Geometry check sheet. Reference: the model listing, model coordinates, mm. Round coordinates to 2 decimals unless told otherwise and drop trailing zeros. Write each loop counter-clockwise with the first axis right and the second up, starting at its lowest first coordinate (ties: lowest second). Pieces come first, ordered by that corner, then holes. Notation, with made-up numbers: M -12,-6.5 L -1,-6.5 A14 cw -1,2.5 Z; hole C 63,-28 d8. An arc over 180 degrees is marked long. Answer in a Markdown table with one row per item. Add a question column.
from build123d import *

# Parameters (mm, degrees)
SKETCH1_R            = 84
BOSS_EXTRUDE1_DEPTH  = 10
M6_CLEARANCE_HOLE1_D = 7


with BuildPart() as part:
    # Sketch1 → Boss-Extrude1 (new body)
    with BuildSketch(Plane(origin=(0, 0, 0), x_dir=(1, 0, 0), z_dir=(0, 1, 0))):
        with Locations(Location((0, 0, 0), (0, 0, 270))):
            Circle(SKETCH1_R)
    extrude(amount=BOSS_EXTRUDE1_DEPTH)

    # M6 Clearance Hole1 (through all)
    with Locations(Plane(origin=(0, 10, -76), x_dir=(0, 0, 1), z_dir=(0, 1, 0))):
        with Locations((0, 0), (76, -76), (76, 76), (76, 25), (51, 0), (76, -25), (101, 0), (152, 0)):
            Hole(M6_CLEARANCE_HOLE1_D / 2)


solid = part.part
Item 1: Section check B-B, the plane x = 0. Record the boundary of the cut face in (y, z).
Item 2: Section check C-C, the plane y = 3. Give the number of separate pieces and of enclosed holes in the cut face, and give its area (3 significant figures).
Item 3: Section check D-D, the plane x = 76. Record the boundary of the cut face in (y, z), and give its area (3 significant figures).
Item 4: Section check A-A, the plane z = 0. Record the boundary of the cut face in (x, y), and give its area (3 significant figures).
Item 5: Mould release check, pull along X, two halves, no side actions. Record for faces 1 (the cylindrical face through (25.23, 4.93, 80.12)), 2 (the cylindrical face through (-21.53, 4.93, 0.46)), 3 (the flat face through (1, 0, -1)): +X half, -X half, draft (parallel to the pull), parting line (faces both ways), or undercut.
Item 6: Scan lines: probe 1 along Z at (x, y) = (0.5, 6.5); probe 2 along X at (y, z) = (4.75, 0); probe 3 along X at (y, z) = (6.25, -76). Record each from-to range of solid material in increasing order. Write a range as from..to.
Item 7: Gauge pin test, flat ends, axial feed: pin 1 Ø6 at (x, z) = (-23.5, 29) entering from -Y; pin 2 Ø4 at (y, z) = (1.5, 27) entering from +X; pin 3 Ø1.5 at (y, z) = (6, 35) entering from -X. Record the tip position at first contact, or that the pin passes through.
Result sheet:
| question | item | result |
|---|---|---|
| 1 | outline | M 0,-84 L 10,-84 L 10,-79.5 L 0,-79.5 Z; M 0,-72.5 L 10,-72.5 L 10,-28.5 L 0,-28.5 Z; M 0,-21.5 L 10,-21.5 L 10,21.5 L 0,21.5 Z; M 0,28.5 L 10,28.5 L 10,72.5 L 0,72.5 Z; M 0,79.5 L 10,79.5 L 10,84 L 0,84 Z |
| 2 | separate pieces | 1 |
| 2 | enclosed holes | 8 |
| 2 | area | 21,900 mm^2 |
| 3 | outline | M 0,-35.78 L 10,-35.78 L 10,-3.5 L 0,-3.5 Z; M 0,3.5 L 10,3.5 L 10,35.78 L 0,35.78 Z |
| 3 | area | 646 mm^2 |
| 4 | outline | M -84,0 L -79.5,0 L -79.5,10 L -84,10 Z; M -72.5,0 L -28.5,0 L -28.5,10 L -72.5,10 Z; M -21.5,0 L 21.5,0 L 21.5,10 L -21.5,10 Z; M 28.5,0 L 72.5,0 L 72.5,10 L 28.5,10 Z; M 79.5,0 L 84,0 L 84,10 L 79.5,10 Z |
| 4 | area | 1,400 mm^2 |
| 5 | face 1 | parting line |
| 5 | face 2 | undercut |
| 5 | face 3 | draft |
| 6 | probe 1 | z = -84..-79.46, -72.54..-28.46, -21.54..21.54, 28.46..72.54, 79.46..84 |
| 6 | probe 2 | x = -84..-79.5, -72.5..-28.5, -21.5..21.5, 28.5..72.5, 79.5..84 |
| 6 | probe 3 | x = -35.78..-3.5, 3.5..35.78 |
| 7 | pin 1 | stops at y = 0 |
| 7 | pin 2 | stops at x = 80.19 |
| 7 | pin 3 | stops at x = -76.7 |
